Check sheet for the drawn part. Datum: minimum x, y, z corner. Units: mm. A direction names the side the tool comes from. Give positions to 0.01 mm unless a question says otherwise; leave off trailing zeros. Order: outer loops, then holes, each group sorted by start corner. A loop starts at its lowest first (then second) coordinate and runs counter-clockwise, first axis right, second up. Notation, with made-up numbers: (79.25, 2.5) -> (114.25, 2.5) arc R21 ccw to (114.25, 22.5) -> close; hole circle Ø2 at (54, 58). An arc over 180 degrees is marked (long way). Answer in a Markdown table with one row per item. Add a question column.
(1) Cross-section at D-D (y = 25). Record the cut outline in (x, z), then the cut area to 3 significant figures.
(2) Thickness scan on L1, parallel to Z at x = 36.5, y = 7; L2, parallel to Z at x = 1.45, y = 25; L3, parallel to X at y = 24, z = 34. Record the ranges inside material, lowest first. Write a range as [from, to].
(3) Cross-section at B-B (z = 25). Record the cut outline in (x, y).
(4) Release check for a two-part mould opening along Z. For the marked faces 1, 2 and 3 record: released by +Z, released by -Z, zero draft, split by the parting line, or undercut.
(5) Cross-section at A-A (x = 34). Record the cut outline in (y, z).
(6) Go/stop test with flat-tipped pins: pin 1 (5 mm diameter, centred on y = 39, z = 18.5, fed in from +X); pin 2 (7 mm diameter, centred on y = 25, z = 25, fed in from -X). Record where each tip stops, or that it passes through.
(7) Cross-section at C-C (y = 30.5). Record the cut outline in (x, z).
(8) Set-up check for the marked faces 4 and 5: record each of +Z, -Z, +X, -X, +Y, -Y from which the full face is reachable in a straight line by a thin tool's end or side.
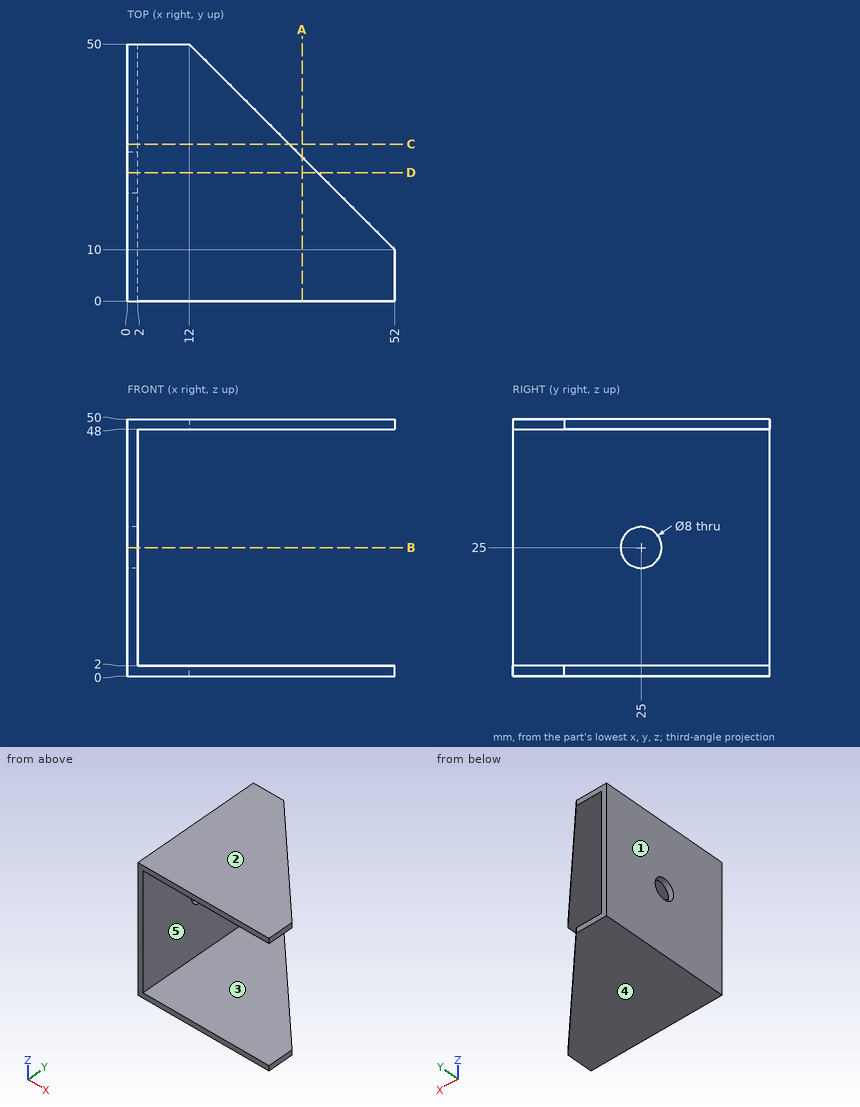
Answer below:
| question | item | result |
|---|---|---|
| 1 | outline | (0, 0) -> (37, 0) -> (37, 2) -> (2, 2) -> (2, 21) -> (0, 21) -> close; (0, 29) -> (2, 29) -> (2, 48) -> (37, 48) -> (37, 50) -> (0, 50) -> close |
| 1 | area | 224 mm² |
| 2 | L1 | z = [0, 2], [48, 50] |
| 2 | L2 | z = [0, 21], [29, 50] |
| 2 | L3 | x = [0, 2] |
| 3 | outline | (0, 0) -> (2, 0) -> (2, 21) -> (0, 21) -> close; (0, 29) -> (2, 29) -> (2, 50) -> (0, 50) -> close |
| 4 | face 1 | zero draft |
| 4 | face 2 | released by +Z |
| 4 | face 3 | undercut |
| 5 | outline | (0, 0) -> (28, 0) -> (28, 2) -> (0, 2) -> close; (0, 48) -> (28, 48) -> (28, 50) -> (0, 50) -> close |
| 6 | pin 1 | stops at x = 2 |
| 6 | pin 2 | passes through |
| 7 | outline | (0, 0) -> (31.5, 0) -> (31.5, 2) -> (2, 2) -> (2, 48) -> (31.5, 48) -> (31.5, 50) -> (0, 50) -> close |
| 8 | face 4 | -Z, +X, -X, +Y, -Y |
| 8 | face 5 | +X, +Y, -Y |
